```python
from build123d import *

# Parameters (mm, degrees)
F0_R        = 15.7049958866
F1_DEPTH    = 10
F2_R        = 5.08
F3_T2_ANGLE = 138.8894896051


# Not quite as in the source:
# - a fillet or chamfer that OpenCascade refuses, or shapes differently, is made with other operations: its cross-section is extruded or revolved along the edge and cut away or added


with BuildPart() as f1:
    # F0 (on Top) → F1 (new body)
    with BuildSketch(Plane.XY):
        with BuildLine():
            Line((-67.6743760705, 33.6404591799), (-67.6743760705, -30.8862738311))
            Line((-67.6743760705, -30.8862738311), (72.3958462477, -30.8862738311))
            Line((72.3958462477, -30.8862738311), (72.3958462477, 33.6404591799))
            ThreePointArc((72.3958462477, 33.6404591799), (2.3607350886, 74.4084313611), (-67.6743760705, 33.6404591799))
        make_face()
        Circle(F0_R, mode=Mode.SUBTRACT)
    extrude(amount=F1_DEPTH)

    # F2
    f2_edges = [f1.edges().sort_by_distance(p)[0] for p in [
        (2.360735, 74.408431, 10),
    ]]
    fillet(f2_edges, radius=F2_R)

    # F3: fillet of radius 5.08 on 1 edges, made by hand

    # F3_s1 → F3_t2 (revolve, cut)
    with BuildSketch(Plane(origin=(2.3069814419, -6.152208534, 0), x_dir=(0, 0, 1), z_dir=(0.351110531, -0.9363340189, 0))):
        with BuildLine():
            ThreePointArc((4.92, -80.5978917459), (1.4317675513, -79.0554933848), (0, -75.5204120561))
            Line((0, -75.5204120561), (0, -80.5978917459))
            Line((0, -80.5978917459), (4.92, -80.5978917459))
        make_face()
    revolve(axis=Axis((2.3607350886, -6.1320517619, 0), (0, 0, 1)), revolution_arc=F3_T2_ANGLE, mode=Mode.SUBTRACT)


solid = f1.part
```
Geometry: final body of the model. Coordinates: model frame, mm. Round coordinates to 2 decimals unless told otherwise and drop trailing zeros. Write each loop counter-clockwise with the first axis right and the second up, starting at its lowest first coordinate (ties: lowest second). Pieces come first, ordered by that corner, then holes. Notation, with made-up numbers: (84.5, 25.25) -> (138.5, 25.25) arc R6 cw to (138.5, 36.25) -> close; hole circle Ø9 at (-12.75, 8.5). An arc over 180 degrees is marked (long way). Return JSON: item names as keys, results as strings.
Q1. Section C-C on y = -11. Return the cut outline in (x, z).
From the geometry:
{"outline": "(-67.67, 0) -> (-11.21, 0) -> (-11.21, 10) -> (-67.67, 10) -> close; (11.21, 0) -> (72.4, 0) -> (72.4, 10) -> (11.21, 10) -> close"}
Q2. Ray query, line 1 (X direction, y = 3.5, z = 5.5); line 2 (Y direction, x = 0, z = 7.5) (3 decimals); line 3 (Y direction, x = 0, z = 2.25) (3 decimals). Return the intervals inside material, ascending.
From the geometry:
{"line 1": "-67.67 to -15.31, 15.31 to 72.4", "line 2": "-30.886 to -15.705, 15.705 to 73.67", "line 3": "-30.886 to -15.705, 15.705 to 73.515"}
Q3. First-contact query: pin 1 Ø4 at (x, z) = (-30, 1) entering from +Y. Flat tip, straight axial feed; report the tip coordinate or a pass-through.
From the geometry:
{"pin 1": "y = 67.44"}
Q4. Section B-B on z = 1.75. Return the cut outline in (x, y) (3 decimals), and give its area (3 significant figures).
From the geometry:
{"outline": "(-67.674, -30.886) -> (72.396, -30.886) -> (72.396, 31.063) arc R79.299 ccw to (-67.674, 31.063) -> close; hole circle Ø31.41 at (0, 0)", "area": "12,100 mm2"}
Q5. Mould query, pull axis X, two halves, no side actions, for faces 1 (the cylindrical face through (14.98, 4.72, 4.93)), 2 (the flat face through (1, 20, 0)), 3 (the flat face through (72.396, 1, 5)). Classes: +X half, -X half, draft (parallel to the pull), parting line (faces both ways), or undercut.
From the geometry:
{"face 1": "undercut", "face 2": "draft", "face 3": "+X half"}
Q6. Section A-A on y = 0. Return the cut outline in (x, z) (3 decimals), and give its area (3 significant figures).
From the geometry:
{"outline": "(-67.674, 0) -> (-15.705, 0) -> (-15.705, 10) -> (-67.674, 10) -> close; (15.705, 0) -> (72.396, 0) -> (72.396, 10) -> (15.705, 10) -> close", "area": "1,090 mm2"}
